Input: part model. Units: mm. Frame: model coordinates. A direction names the side the tool comes from. Coordinates: 2 decimals unless noted, no trailing zeros. Loops run counter-clockwise (first coordinate to the right, second up) from the corner with the lowest first, then second, coordinate; pieces in that order, holes last. Notation, with made-up numbers: (-27.5, 57.5) -> (29.5, 57.5) arc R12 cw to (29.5, 61.5) -> close; hole circle Ø9 at (74.25, 89). An arc over 180 degrees is marked (long way). Answer as a JSON object with one key per item and string values.
from build123d import *

# Parameters (mm, degrees)
F1_DEPTH = 44.45
F2_W     = 28.3845
F2_H     = 63.4492
F3_DEPTH = 114.3
F5_DEPTH = 127
F6_R     = 5.08


with BuildPart() as f1:
    # F0 (on Front) → F1 (new body)
    with BuildSketch(Plane.XZ):
        with BuildLine():
            Line((0, 83.82), (0, 0))
            Line((0, 0), (114.3, 0))
            Line((114.3, 0), (114.3, 83.82))
            Line((114.3, 83.82), (101.6, 83.82))
            Line((101.6, 83.82), (101.6, 60.7949))
            ThreePointArc((101.6, 60.7949), (57.15, 16.3449), (12.7, 60.7949))
            Line((12.7, 60.7949), (12.7, 83.82))
            Line((12.7, 83.82), (0, 83.82))
        make_face()
    extrude(amount=-F1_DEPTH)

    # F2 (on face) → F3 (cut)
    with BuildSketch(Plane.YZ.offset(114.3)):
        with Locations((30.25775, 52.0954)):
            Rectangle(F2_W, F2_H)
    extrude(amount=-F3_DEPTH, mode=Mode.SUBTRACT)

    # F4 (on face) → F5 (cut)
    with BuildSketch(Plane.XZ):
        with BuildLine():
            Line((0, 16.3449), (57.15, 16.3449))
            ThreePointArc((57.15, 16.3449), (25.7191035763, 29.3640035763), (12.7, 60.7949))
            Line((12.7, 60.7949), (12.7, 83.82))
            Line((12.7, 83.82), (0, 83.82))
            Line((0, 83.82), (0, 16.3449))
        make_face()
    extrude(amount=-F5_DEPTH, mode=Mode.SUBTRACT)

    # F6
    f6_edges = [f1.edges().sort_by_distance(p)[0] for p in [
        (107.95, 0, 83.82),
        (101.6, 8.03275, 83.82),
        (107.95, 16.0655, 83.82),
        (114.3, 8.03275, 83.82),
    ]]
    fillet(f6_edges, radius=F6_R)


solid = f1.part
1. Pin query (flat end, axial travel): P1, Ø6, axis at x = 33, y = 27.5, coming from the +Z side; P2, Ø8, axis at y = 8.5, z = 64.5, coming from the -X side; P3, Ø4, axis at x = 29, y = 4.5, coming from the -Z side; P4, Ø1, axis at x = 63.5, y = 39.5, coming from the +Z side. Return the tip coordinate at first contact, or that it passes through.
Reply:
{"P1": "stops at z = 16.34", "P2": "stops at x = 101.6", "P3": "stops at z = 0", "P4": "stops at z = 16.88"}
2. Access query for faces 1 (the face through (101.6, 8, 70)), 2 (the face through (104, 16.066, 43)), 3 (the face through (113.35, 8.15, 81.7)). Directions: +Z, -Z, +X, -X, +Y, -Y. A direction counts if a zero-diameter tool reaches every point of the face in a straight line with its end or side. Return the directions, or none.
Reply:
{"face 1": "+Z, -X, +Y, -Y", "face 2": "+Z, +X, -X, +Y", "face 3": "+Z, +X, +Y, -Y"}
3. Section query C-C (x = 53.5). Return loops of the section in (y, z), plus the area to 3 significant figures.
Reply:
{"outline": "(0, 0) -> (44.45, 0) -> (44.45, 16.34) -> (0, 16.34) -> close", "area": "727 mm2"}
4. Section query A-A (y = 26.5). Return loops of the section in (x, z), plus the area to 3 significant figures.
Reply:
{"outline": "(0, 0) -> (114.3, 0) -> (114.3, 20.37) -> (75.63, 20.37) arc R44.45 cw to (57.15, 16.34) -> (0, 16.34) -> close", "area": "2,050 mm2"}
5. Section query D-D (y = 3). Return loops of the section in (x, z), plus the area to 3 significant figures.
Reply:
{"outline": "(0, 0) -> (114.3, 0) -> (114.3, 78.74) arc R5.08 ccw to (111.3, 83.37) -> (104.6, 83.37) arc R5.08 ccw to (101.6, 78.74) -> (101.6, 60.79) arc R44.45 cw to (57.15, 16.34) -> (0, 16.34) -> close", "area": "3,140 mm2"}
6. Line query: line 1 along Z through (x, y) = (9.5, 15); line 2 along Z through (x, y) = (77, 24); line 3 along Y through (x, z) = (93, 23). Output: solid intervals per line, ascending.
Reply:
{"line 1": "z = 0 to 16.34", "line 2": "z = 0 to 20.37", "line 3": "y = 0 to 16.07"}
7. Section query B-B (z = 67.5). Return loops of the section in (x, y), plus the area to 3 significant figures.
Reply:
{"outline": "(101.6, 0) -> (114.3, 0) -> (114.3, 16.07) -> (101.6, 16.07) -> close", "area": "204 mm2"}
